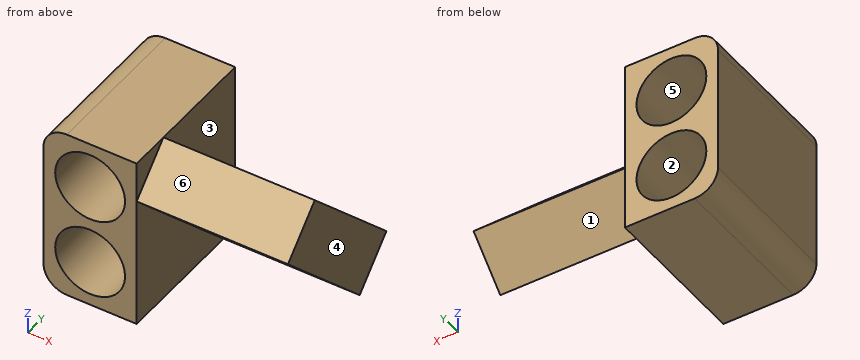
Autodesk Inventor part; units mm, degrees
ref_plane "YZ Plane" through (0, 0, 0) normal (1, 0, 0) x (0, 1, 0)
ref_plane "XZ Plane" through (0, 0, 0) normal (0, 1, 0) x (-1, 0, 0)
ref_plane "XY Plane" through (0, 0, 0) normal (0, 0, 1) x (1, 0, 0)
sketch "Szkic1" plane through (0, 0, 0) normal (0, 1, 0) x (-1, 0, 0)
  circle A0 centre (-0.3368, -8.6859) radius 3
  circle A1 centre (-0.3368, -1.6859) radius 3
  line L0 (3.6632, 2.3141) -> (-4.3368, 2.3141)
  line L1 (-4.3368, 2.3141) -> (-4.3368, -12.6859)
  line L2 (-4.3368, -12.6859) -> (3.6632, -12.6859)
  line L3 (3.6632, -12.6859) -> (3.6632, 2.3141)
  point P0 (0, 0)
  dimension "d0" = 6
  dimension "d1" = 6
  dimension "d2" = 7
  dimension "d3" = 8
  dimension "d4" = 15
  dimension "d5" = 4
  dimension "d6" = 4
extrude "Wyciągnięcie proste1" add sketch "Szkic1" along normal blind 13
fillet "Zaokrąglenie1" radius 2 2 edges at (-3.6632, 6.5, 2.3141) (-3.6632, 6.5, -12.6859)
sketch "Szkic2" plane through (4.3368, 0, 0.3141) normal (1, 0, 0) x (0, 0, -1)
  line L0 (6, 13) -> (6, 0) construction
  line L1 (-2, 0) -> (13, 0)
  line L2 (13, 0) -> (13, 13)
  line L3 (-2, 13) -> (13, 13)
  line L4 (-2, 0) -> (-2, 13)
  line L5 (-2, 3.5355) -> (1.5355, 0)
  line L6 (-2, 3.5355) -> (3, 3.5355) construction
  line L7 (1.5355, 0) -> (11, 9.4645)
  line L8 (11, 9.4645) -> (7.4645, 13)
  line L9 (7.4645, 13) -> (-2, 3.5355)
  line L10 (-2, 0) -> (-2, 13) construction
  dimension "d18" = 45
  dimension "d19" = 90
  dimension "d20" = 90
  dimension "d21" = 5
extrude "Wyciągnięcie proste2" add sketch "Szkic2" along normal blind 13 and the other way blind 1 contours L5 L9 L8 L7
properties part number "obudowa_stand"
Work out the finished part from the listing and answer in its coordinate system (mm). Face numbers are marked on the shaded views. A direction names the side the tool comes from. Give positions to 0.01 mm unless a question says otherwise; leave off trailing zeros. Write each loop counter-clockwise with the first axis right and the second up, starting at its lowest first coordinate (ties: lowest second). Pieces come first, ordered by that corner, then holes.
(1) The part is cut by section D-D on x = 9. Write down the section's boundary in (y, z).
Final values:
outline: (0, -1.22) - (9.46, -10.69) - (13, -7.15) - (3.54, 2.31) - close
(2) The part is cut by section C-C on y = 1. Write down the section's boundary in (x, z), plus the area to 3 significant figures.
Final values:
outline: (-3.66, -10.69) arc R2 ccw to (-1.66, -12.69) - (4.34, -12.69) - (4.34, -2.22) - (17.34, -2.22) - (17.34, -0.22) - (4.34, -0.22) - (4.34, 2.31) - (-1.66, 2.31) arc R2 ccw to (-3.66, 0.31) - close; hole circle Ø6 at (0.34, -8.69); hole circle Ø6 at (0.34, -1.69)
area: 87.7 mm2
(3) The mould has two halves that part along Z. Classify the marked faces 4, 5 and 6: pulls with the +Z half, pulls with the -Z half, needs draft (parallel to the pull), parting line crosses it, or undercut.
Final values:
face 4: needs draft
face 5: undercut
face 6: pulls with the +Z half
(4) The part is cut by section B-B on x = -2. Write down the section's boundary in (y, z).
Final values:
outline: (0, -12.66) - (13, -12.66) - (13, -10.57) - (0, -10.57) - close; (0, -6.8) - (13, -6.8) - (13, -3.57) - (0, -3.57) - close; (0, 0.2) - (13, 0.2) - (13, 2.29) - (0, 2.29) - close
(5) Flat-ended cylindrical pins translate along their axes: pin 1 Ø1.5 at (x, y) = (9, 5) entering from -Z; pin 2 Ø5 at (x, y) = (12, 5.5) entering from +Z; pin 3 Ø3 at (y, z) = (2.5, -9) entering from +X. Find the tip coordinate at first contact, or state that the pin passes through.
Final values:
pin 1: stops at z = -6.97
pin 2: stops at z = 2.31
pin 3: stops at x = 4.34
(6) The part is cut by section A-A on z = -6.25. Write down the section's boundary in (x, y), plus the area to 3 significant figures.
Final values:
outline: (-3.66, 0) - (-1.41, 0) - (-1.41, 13) - (-3.66, 13) - close; (2.09, 0) - (4.34, 0) - (4.34, 5.03) - (17.34, 5.03) - (17.34, 12.1) - (4.34, 12.1) - (4.34, 13) - (2.09, 13) - close
area: 150 mm2
(7) Straight lines are drawn through the part: line 1 (Z direction, x = 1.25, y = 11); line 2 (X direction, y = 9, z = -8.5); line 3 (Z direction, x = -1, y = 2). For each, find the intervals that lie inside material, in ascending order.
Final values:
line 1: z = -12.69 to -11.54, -5.83 to -4.54, 1.17 to 2.31
line 2: x = -3.66 to -2.66, 3.33 to 17.34
line 3: z = -12.69 to -11.37, -6 to -4.37, 1 to 2.31
(8) Which of the six approach directions +Z, -Z, +X, -X, +Y, -Y give full straight-line access (tool end or side, diameter ignored) to the marked faces 1, 2 and 3?
Final values:
face 1: -Z, +X, +Y
face 2: +Y, -Y
face 3: +Z, +X, +Y
